Here's how the part is built. I have some questions about the finished solid (model axes, mm). Round coordinates to 2 decimals unless told otherwise and drop trailing zeros. Write each loop counter-clockwise with the first axis right and the second up, starting at its lowest first coordinate (ties: lowest second). Pieces come first, ordered by that corner, then holes. Notation, with made-up numbers: (59, 48.5) -> (101, 48.5) arc R30 ccw to (101, 83.5) -> close; hole circle Ø4 at (32, 33). An arc over 180 degrees is marked (long way). Put each result on its own line as item: value. Start each with the question number.
1. Suppose I cut it at A-A (x = 22.3). Please give me the cut outline in (y, z).
2. Suppose I cut it at D-D (z = 1.8). Count the separate pieces of the cut face and the enclosed holes in it, then the cut area to 3 significant figures.
3. Suppose I cut it at B-B (x = 1). Please give me the cut outline in (y, z).
4. I need wall thicknesses on probe 1 along Y at (x, z) = (-22, 1.1); probe 2 along Y at (x, z) = (-10, 0.7); probe 3 along Y at (x, z) = (0, 1). Which ranges of each line are inside material? Lowest first, please. Write a range as from..to.
5. For pin 1 (4.5 mm diameter, centred on x = 0, y = -22.3, fed in from -Z), with a flat end and sliding along its axis, tell me the tip position at first contact or that it passes through.
6. Suppose I cut it at C-C (y = -10). Please give me the cut outline in (x, z).
```python
from build123d import *

# Parameters (mm, degrees)
SKETCH1_W           = 80
SKETCH1_H           = 80
SKETCH1_R           = 2.6
SKETCH1_R_2         = 3.55
BOSS_EXTRUDE1_DEPTH = 3.2
FILLET1_R           = 10


with BuildPart() as part:
    # Sketch1 → Boss-Extrude1 (new body)
    with BuildSketch(Plane.XY):
        Rectangle(SKETCH1_W, SKETCH1_H)
        Circle(SKETCH1_R, mode=Mode.SUBTRACT)
        with Locations((0, 10)):
            Circle(SKETCH1_R, mode=Mode.SUBTRACT)
        with Locations((0, 22.3)):
            Circle(SKETCH1_R, mode=Mode.SUBTRACT)
        with Locations((0, -10)):
            Circle(SKETCH1_R, mode=Mode.SUBTRACT)
        with Locations((0, -22.3)):
            Circle(SKETCH1_R, mode=Mode.SUBTRACT)
        with Locations((10, 0)):
            Circle(SKETCH1_R, mode=Mode.SUBTRACT)
        with Locations((-10, 0)):
            Circle(SKETCH1_R, mode=Mode.SUBTRACT)
        with Locations((-22.3, 0)):
            Circle(SKETCH1_R_2, mode=Mode.SUBTRACT)
        with Locations((22.3, 0)):
            Circle(SKETCH1_R, mode=Mode.SUBTRACT)
        with Locations((22.3, 22.3)):
            Circle(SKETCH1_R, mode=Mode.SUBTRACT)
        with Locations((22.3, -22.3)):
            Circle(SKETCH1_R, mode=Mode.SUBTRACT)
        with Locations((-22.3, -22.3)):
            Circle(SKETCH1_R_2, mode=Mode.SUBTRACT)
        with Locations((-22.3, 22.3)):
            Circle(SKETCH1_R_2, mode=Mode.SUBTRACT)
    extrude(amount=BOSS_EXTRUDE1_DEPTH)

    # Fillet1
    fillet1_edges = [part.edges().sort_by_distance(p)[0] for p in [
        (40, -40, 1.6),
        (-40, -40, 1.6),
        (-40, 40, 1.6),
        (40, 40, 1.6),
    ]]
    fillet(fillet1_edges, radius=FILLET1_R)


solid = part.part
```
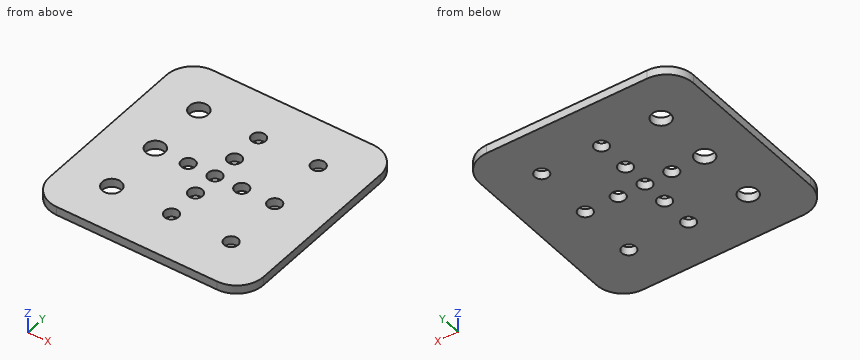
Verdict:
1. outline: (-40, 0) -> (-24.9, 0) -> (-24.9, 3.2) -> (-40, 3.2) -> close; (-19.7, 0) -> (-2.6, 0) -> (-2.6, 3.2) -> (-19.7, 3.2) -> close; (2.6, 0) -> (19.7, 0) -> (19.7, 3.2) -> (2.6, 3.2) -> close; (24.9, 0) -> (40, 0) -> (40, 3.2) -> (24.9, 3.2) -> close
2. separate pieces: 1
2. enclosed holes: 13
2. area: 5,980 mm^2
3. outline: (-40, 0) -> (-24.7, 0) -> (-24.7, 3.2) -> (-40, 3.2) -> close; (-19.9, 0) -> (-12.4, 0) -> (-12.4, 3.2) -> (-19.9, 3.2) -> close; (-7.6, 0) -> (-2.4, 0) -> (-2.4, 3.2) -> (-7.6, 3.2) -> close; (2.4, 0) -> (7.6, 0) -> (7.6, 3.2) -> (2.4, 3.2) -> close; (12.4, 0) -> (19.9, 0) -> (19.9, 3.2) -> (12.4, 3.2) -> close; (24.7, 0) -> (40, 0) -> (40, 3.2) -> (24.7, 3.2) -> close
4. probe 1: y = -40..-25.84, -18.76..-3.54, 3.54..18.76, 25.84..40
4. probe 2: y = -40..-2.6, 2.6..40
4. probe 3: y = -40..-24.9, -19.7..-12.6, -7.4..-2.6, 2.6..7.4, 12.6..19.7, 24.9..40
5. pin 1: passes through
6. outline: (-40, 0) -> (-2.6, 0) -> (-2.6, 3.2) -> (-40, 3.2) -> close; (2.6, 0) -> (40, 0) -> (40, 3.2) -> (2.6, 3.2) -> close
